Could you check a few things on this model? Use its own coordinates, in mm. A direction names the side the tool comes from. Give positions to 0.01 mm unless a question says otherwise; leave off trailing zeros. Loops run counter-clockwise (first coordinate to the right, second up) from the corner with the lowest first, then second, coordinate; pieces in that order, holes last. Notation, with made-up numbers: (-18, 78) - (29, 78) arc R13 ccw to (29, 85) - close; hole circle Ø11 at (15.5, -37). An arc over 180 degrees is marked (long way). Write each question's results on one line, items separated by ' | '. Start each with the question number.
1) I'm going to push a flat-ended pin straight in: pin 1 (4 mm diameter, centred on x = 54, z = -75, fed in from +Y). Where does the tip first touch, or does it pass through?
2) I want a section at B-B, the plane y = 3. Count the separate pieces of the cut face and the enclosed holes in it, and give its area (3 significant figures).
3) On a 3-axis mill with a long thin cutter (end or side, diameter ignored), from which of +Z, -Z, +X, -X, +Y, -Y can I reach the whole of each face in a straight line? I mean faces 1 (the face through (70, 2, 1)), 2 (the face through (34.67, 7.75, 82.52)), 3 (the face through (-59, 3, 75)). Say none if no direction works.
4) I want a section at A-A, the plane z = 63. Write out the boundary of the cut face in (x, y), and give its area (3 significant figures).
5) If we mould it in two halves opening along Z, with no side actions, what happens to faces 4 (the face through (-10.415, 2.535, 11.829)), 5 (the face through (36, 8, 56))? For each: +Z half, -Z half, draft (parallel to the pull), parting line (faces both ways), or undercut.
6) If I drill on probe 1 along Z at (x, y) = (46.5, 2.55); probe 2 along Z at (x, y) = (-46.5, 3.3); probe 3 along X at (y, z) = (1, 40), over which ranges is the centre line in solid material (lowest first)? Write a range as [from, to].
from build123d import *

# Parameters (mm, degrees)
SKETCH1_W           = 140
SKETCH1_H           = 190
SKETCH1_R           = 2.5
BOSS_EXTRUDE1_DEPTH = 5
FILLET1_R           = 10
SKETCH3_R           = 1.5
CUT_EXTRUDE2_DEPTH  = 10
SKETCH14_W          = 12.5
SKETCH14_H          = 150
CUT_EXTRUDE9_DEPTH  = 10
FILLET3_R           = 2
SKETCH17_R          = 2.5
CUT_EXTRUDE12_DEPTH = 10
SKETCH18_R          = 2.5
SKETCH18_R_2        = 1.5
BOSS_EXTRUDE2_DEPTH = 3
CUT_EXTRUDE13_DEPTH = 6
CHAMFER1_SIZE       = 2.5


with BuildPart() as part:
    # Sketch1 → Boss-Extrude1 (new body)
    with BuildSketch(Plane(origin=(0, 0, 0), x_dir=(1, 0, 0), z_dir=(0, 1, 0))):
        Rectangle(SKETCH1_W, SKETCH1_H)
        with Locations((60, -89)):
            Circle(SKETCH1_R, mode=Mode.SUBTRACT)
        with Locations((60, 89)):
            Circle(SKETCH1_R, mode=Mode.SUBTRACT)
        with Locations((-60, 89)):
            Circle(SKETCH1_R, mode=Mode.SUBTRACT)
        with Locations((-60, -89)):
            Circle(SKETCH1_R, mode=Mode.SUBTRACT)
    extrude(amount=BOSS_EXTRUDE1_DEPTH)

    # Fillet1
    fillet1_edges = [part.edges().sort_by_distance(p)[0] for p in [
        (-70, 2.5, 95),
        (-70, 2.5, -95),
        (70, 2.5, -95),
        (70, 2.5, 95),
    ]]
    fillet(fillet1_edges, radius=FILLET1_R)

    # Sketch3 → Cut-Extrude2 (cut)
    with BuildSketch(Plane(origin=(0, 5, 0), x_dir=(1, 0, 0), z_dir=(0, 1, 0))):
        with Locations((4.5, -54.5)):
            Circle(SKETCH3_R)
        with Locations((35, -54.5)):
            Circle(SKETCH3_R)
        with Locations((4.5, -85)):
            Circle(SKETCH3_R)
        with Locations((35, -85)):
            Circle(SKETCH3_R)
    extrude(amount=-CUT_EXTRUDE2_DEPTH, mode=Mode.SUBTRACT)

    # Sketch14 → Cut-Extrude9 (cut)
    with BuildSketch(Plane(origin=(0, 5, 0), x_dir=(1, 0, 0), z_dir=(0, 1, 0))):
        with Locations((-58.75, 0)):
            Rectangle(SKETCH14_W, SKETCH14_H)
        with Locations((58.75, 0)):
            Rectangle(SKETCH14_W, SKETCH14_H)
        Polygon((-35, -49.5), (-10, -49.5), (-10, -90), (-35, -90), (-35, -73.5), (-50, -73.5), (-50, -49.5), align=None)
        with BuildLine():
            Line((-35.5, 89.3), (35.5, 89.3))
            ThreePointArc((35.5, 89.3), (36.914213562, 88.714213562), (37.5, 87.3))
            Line((37.5, 87.3), (37.5, 76.5))
            ThreePointArc((37.5, 76.5), (36.914213562, 75.085786438), (35.5, 74.5))
            Line((35.5, 74.5), (-35.5, 74.5))
            ThreePointArc((-35.5, 74.5), (-36.914213562, 75.085786438), (-37.5, 76.5))
            Line((-37.5, 76.5), (-37.5, 87.3))
            ThreePointArc((-37.5, 87.3), (-36.914213562, 88.714213562), (-35.5, 89.3))
        make_face()
        Polygon((-24.5, -23.085786438), (-1.414213562, 0), (-24.5, 23.085786438), align=None)
        Polygon((23.085786438, 24.5), (-23.085786438, 24.5), (0, 1.414213562), align=None)
        Polygon((24.5, -23.085786438), (24.5, 23.085786438), (1.414213562, 0), align=None)
        Polygon((-23.085786438, -24.5), (23.085786438, -24.5), (0, -1.414213562), align=None)
    extrude(amount=-CUT_EXTRUDE9_DEPTH, mode=Mode.SUBTRACT)

    # Fillet3
    fillet3_edges = [part.edges().sort_by_distance(p)[0] for p in [
        (-65, 2.5, 75),
        (-65, 2.5, -75),
        (-52.5, 2.5, -75),
        (-52.5, 2.5, 75),
        (1.414213562, 2.5, 0),
        (24.5, 2.5, -23.085786438),
        (24.5, 2.5, 23.085786438),
        (0, 2.5, -1.414213562),
        (-23.085786438, 2.5, -24.5),
        (23.085786438, 2.5, -24.5),
        (0, 2.5, 1.414213562),
        (23.085786438, 2.5, 24.5),
        (-23.085786438, 2.5, 24.5),
        (-50, 2.5, 49.5),
        (-10, 2.5, 49.5),
        (-10, 2.5, 90),
        (-35, 2.5, 90),
        (-35, 2.5, 73.5),
        (-50, 2.5, 73.5),
        (65, 2.5, -75),
        (65, 2.5, 75),
        (52.5, 2.5, 75),
        (52.5, 2.5, -75),
        (-24.5, 2.5, 23.085786438),
        (-24.5, 2.5, -23.085786438),
        (-1.414213562, 2.5, 0),
    ]]
    fillet(fillet3_edges, radius=FILLET3_R)

    # Sketch17 → Cut-Extrude12 (cut)
    with BuildSketch(Plane(origin=(0, 5, 0), x_dir=(1, 0, 0), z_dir=(0, 1, 0))):
        with Locations((46.5, 85)):
            Circle(SKETCH17_R)
        with Locations((46.5, -85)):
            Circle(SKETCH17_R)
        with Locations((-46.5, -85)):
            Circle(SKETCH17_R)
        with Locations((-46.5, 85)):
            Circle(SKETCH17_R)
    extrude(amount=-CUT_EXTRUDE12_DEPTH, mode=Mode.SUBTRACT)

    # Sketch18 → Boss-Extrude2 (add)
    with BuildSketch(Plane(origin=(0, 5, 0), x_dir=(1, 0, 0), z_dir=(0, 1, 0))):
        with Locations((4.5, -54.5)):
            Circle(SKETCH18_R)
        with Locations((4.5, -54.5)):
            Circle(SKETCH18_R_2, mode=Mode.SUBTRACT)
        with Locations((35, -54.5)):
            Circle(SKETCH18_R)
        with Locations((35, -54.5)):
            Circle(SKETCH18_R_2, mode=Mode.SUBTRACT)
        with Locations((35, -85)):
            Circle(SKETCH18_R)
        with Locations((35, -85)):
            Circle(SKETCH18_R_2, mode=Mode.SUBTRACT)
        with Locations((4.5, -85)):
            Circle(SKETCH18_R)
        with Locations((4.5, -85)):
            Circle(SKETCH18_R_2, mode=Mode.SUBTRACT)
    extrude(amount=BOSS_EXTRUDE2_DEPTH)

    # Sketch19 → Cut-Extrude13 (cut, through all)
    with BuildSketch(Plane(origin=(0, 5, 0), x_dir=(1, 0, 0), z_dir=(0, 1, 0))):
        with BuildLine():
            Line((-48, -47), (-12, -47))
            ThreePointArc((-12, -47), (-10.585786438, -46.414213562), (-10, -45))
            Line((-10, -45), (-10, -29))
            ThreePointArc((-10, -29), (-10.585786438, -27.585786438), (-12, -27))
            Line((-12, -27), (-48, -27))
            ThreePointArc((-48, -27), (-49.414213562, -27.585786438), (-50, -29))
            Line((-50, -29), (-50, -45))
            ThreePointArc((-50, -45), (-49.414213562, -46.414213562), (-48, -47))
        make_face()
        with BuildLine():
            Line((50, -45), (50, -29))
            ThreePointArc((50, -29), (49.414213562, -27.585786438), (48, -27))
            Line((48, -27), (12, -27))
            ThreePointArc((12, -27), (10.585786438, -27.585786438), (10, -29))
            Line((10, -29), (10, -45))
            ThreePointArc((10, -45), (10.585786438, -46.414213562), (12, -47))
            Line((12, -47), (48, -47))
            ThreePointArc((48, -47), (49.414213562, -46.414213562), (50, -45))
        make_face()
        with BuildLine():
            Line((-48, -24.5), (-29, -24.5))
            ThreePointArc((-29, -24.5), (-27.585786438, -23.914213562), (-27, -22.5))
            Line((-27, -22.5), (-27, 22.5))
            ThreePointArc((-27, 22.5), (-27.585786438, 23.914213562), (-29, 24.5))
            Line((-29, 24.5), (-48, 24.5))
            ThreePointArc((-48, 24.5), (-49.414213562, 23.914213562), (-50, 22.5))
            Line((-50, 22.5), (-50, -22.5))
            ThreePointArc((-50, -22.5), (-49.414213562, -23.914213562), (-48, -24.5))
        make_face()
        with BuildLine():
            Line((48, 24.5), (29, 24.5))
            ThreePointArc((29, 24.5), (27.585786438, 23.914213562), (27, 22.5))
            Line((27, 22.5), (27, -22.5))
            ThreePointArc((27, -22.5), (27.585786438, -23.914213562), (29, -24.5))
            Line((29, -24.5), (48, -24.5))
            ThreePointArc((48, -24.5), (49.414213562, -23.914213562), (50, -22.5))
            Line((50, -22.5), (50, 22.5))
            ThreePointArc((50, 22.5), (49.414213562, 23.914213562), (48, 24.5))
        make_face()
        with BuildLine():
            Line((-40, 66.632125109), (-40, 32.367874891))
            ThreePointArc((-40, 32.367874891), (-38.992955058, 30.631775743), (-36.985959747, 30.644006461))
            Line((-36.985959747, 30.644006461), (-7.861347062, 47.77613157))
            ThreePointArc((-7.861347062, 47.77613157), (-6.875387315, 49.5), (-7.861347062, 51.22386843))
            Line((-7.861347062, 51.22386843), (-36.985959747, 68.355993539))
            ThreePointArc((-36.985959747, 68.355993539), (-38.992955058, 68.368224257), (-40, 66.632125109))
        make_face()
        with BuildLine():
            Line((-26.988652938, 68.27613157), (-1.014040253, 52.996947638))
            ThreePointArc((-1.014040253, 52.996947638), (0, 52.720816068), (1.014040253, 52.996947638))
            Line((1.014040253, 52.996947638), (26.988652938, 68.27613157))
            ThreePointArc((26.988652938, 68.27613157), (27.90434542, 70.525482226), (25.974612685, 72))
            Line((25.974612685, 72), (-25.974612685, 72))
            ThreePointArc((-25.974612685, 72), (-27.90434542, 70.525482226), (-26.988652938, 68.27613157))
        make_face()
        with BuildLine():
            Line((36.985959747, 30.644006461), (7.861347062, 47.77613157))
            ThreePointArc((7.861347062, 47.77613157), (6.875387315, 49.5), (7.861347062, 51.22386843))
            Line((7.861347062, 51.22386843), (36.985959747, 68.355993539))
            ThreePointArc((36.985959747, 68.355993539), (38.992955058, 68.368224257), (40, 66.632125109))
            Line((40, 66.632125109), (40, 32.367874891))
            ThreePointArc((40, 32.367874891), (38.992955058, 30.631775743), (36.985959747, 30.644006461))
        make_face()
        with BuildLine():
            Line((1.014040253, 46.003052362), (26.988652938, 30.72386843))
            ThreePointArc((26.988652938, 30.72386843), (27.90434542, 28.474517774), (25.974612685, 27))
            Line((25.974612685, 27), (-25.974612685, 27))
            ThreePointArc((-25.974612685, 27), (-27.90434542, 28.474517774), (-26.988652938, 30.72386843))
            Line((-26.988652938, 30.72386843), (-1.014040253, 46.003052362))
            ThreePointArc((-1.014040253, 46.003052362), (0, 46.279183932), (1.014040253, 46.003052362))
        make_face()
    extrude(amount=-CUT_EXTRUDE13_DEPTH, mode=Mode.SUBTRACT)

    # Chamfer1
    chamfer1_edges = [part.edges().sort_by_distance(p)[0] for p in [
        (2, 5, 54.5),
        (32.5, 5, 54.5),
        (32.5, 5, 85),
        (2, 5, 85),
    ]]
    chamfer(chamfer1_edges, length=CHAMFER1_SIZE)


solid = part.part
Answers:
1) pin 1: stops at y = 5
2) separate pieces: 1 | enclosed holes: 28 | area: 11,500 mm2
3) face 1: +Z, -Z, +X, +Y, -Y | face 2: +Y | face 3: +Y, -Y
4) outline: (-70, 0) - (-65, 0) - (-65, 5) - (-70, 5) - close; (-52.5, 0) - (-50, 0) - (-50, 5) - (-52.5, 5) - close; (-10, 0) - (52.5, 0) - (52.5, 5) - (-10, 5) - close; (65, 0) - (70, 0) - (70, 5) - (65, 5) - close | area: 375 mm2
5) face 4: undercut | face 5: draft
6) probe 1: z = [-95, -87.5], [-82.5, -24.5], [24.5, 27], [47, 82.5], [87.5, 95] | probe 2: z = [-95, -87.5], [-82.5, -24.5], [24.5, 27], [47, 49.5], [73.5, 82.5], [87.5, 95] | probe 3: x = [-70, -65], [-52.5, -50], [-10, 10], [50, 52.5], [65, 70]
